```python
from build123d import *

# Parameters (mm, degrees)
BOSS_EXTRU_1_DEPTH                           = 6
ESQUISSE2_W                                  = 4
ESQUISSE2_H                                  = 4
BOSS_EXTRU_2_DEPTH                           = 4
TROU_POUR_TARAUDAGE_POUR_TROU_TARAUD_M2_D    = 1.6
TROU_POUR_TARAUDAGE_POUR_TROU_TARAUD_2_REACH = 15.115
TROU_POUR_TARAUDAGE_POUR_TROU_TARAUD_2_B_R   = 0.8
D_GAGEMENT_M31_D                             = 3.6


with BuildPart() as part:
    # Esquisse1 → Boss.-Extru.1 (new body)
    with BuildSketch(Plane.XY):
        Polygon((-10, 4), (10, 4), (10, 0), (7, 0), (7, -2), (2.2, -2), (2.2, 0), (-10, 0), align=None)
    extrude(amount=-BOSS_EXTRU_1_DEPTH)

    # Esquisse2 → Boss.-Extru.2 (add)
    with BuildSketch(Plane.XY):
        with Locations((-8, 2)):
            Rectangle(ESQUISSE2_W, ESQUISSE2_H)
        with Locations((8, 2)):
            Rectangle(ESQUISSE2_W, ESQUISSE2_H)
    extrude(amount=BOSS_EXTRU_2_DEPTH)

    # Trou pour taraudage pour trou taraud_ M2 (through all)
    with Locations(Plane(origin=(10, 0, 0), x_dir=(0, 0, -1), z_dir=(1, 0, 0))):
        with Locations((-2, 2)):
            Hole(TROU_POUR_TARAUDAGE_POUR_TROU_TARAUD_M2_D / 2)

    # Trou pour taraudage pour trou taraud 2 b → Trou pour taraudage pour trou taraud 2 (cut, up to next)
    with BuildSketch(Plane(origin=(0, 4, 0), x_dir=(1, 0, 0), z_dir=(0, 1, 0)), mode=Mode.PRIVATE) as trou_pour_taraudage_pour_trou_taraud_2_sk1:
        with Locations((-8, -2)):
            Circle(TROU_POUR_TARAUDAGE_POUR_TROU_TARAUD_2_B_R)
    trou_pour_taraudage_pour_trou_taraud_2_tool1 = extrude(trou_pour_taraudage_pour_trou_taraud_2_sk1.sketch, amount=-TROU_POUR_TARAUDAGE_POUR_TROU_TARAUD_2_REACH, mode=Mode.PRIVATE) & part.part
    add(trou_pour_taraudage_pour_trou_taraud_2_tool1.solids().sort_by_distance((-8, 4, 2))[0], mode=Mode.SUBTRACT)

    # Dégagement M31 (through all)
    with Locations(Plane(origin=(0, 4, 0), x_dir=(1, 0, 0), z_dir=(0, 1, 0))):
        with Locations((4.6, 3)):
            Hole(D_GAGEMENT_M31_D / 2)


solid = part.part
```
Geometry check sheet. Reference: the model listing, model coordinates, mm. A direction names the side the tool comes from. Give positions to 0.01 mm unless a question says otherwise; leave off trailing zeros. Order: outer loops, then holes, each group sorted by start corner. A loop starts at its lowest first (then second) coordinate and runs counter-clockwise, first axis right, second up.
1. Section check D-D, the plane x = 4.6. Enter the section's corners in (y, z), and give its area (3 significant figures).
2. Access from +Z, -Z, +X, -X, +Y, -Y to the whole of each face (thin tool, end or side, straight path). Record for faces 1 (the face through (-5, 0, -2)), 2 (the face through (7, -1, -3)), 3 (the face through (-7.57, 3.236, 1.325)), 4 (the face through (0, 2, -6)), 5 (the face through (6, 3, 2)).
3. Section check B-B, the plane z = 0.5. Enter the section's corners in (x, y), and give its area (3 significant figures).
4. Release check for a two-part mould opening along X. For faces 6 (the face through (8, 2, 4)), 7 (the face through (1, 2, 0)), 8 (the face through (10, 2, -1)) record: pulls with the +X half, pulls with the -X half, needs draft (parallel to the pull), parting line crosses it, or undercut.
5. Thickness scan on L1, parallel to Z at x = 4.6, y = 0.9; L2, parallel to X at y = 3.2, z = 2.5; L3, parallel to Z at x = -8.8, y = 2. Record the ranges inside material, lowest first.
6. Section check C-C, the plane x = -7. Enter the section's corners in (y, z), and give its area (3 significant figures).
7. Gauge pin test, flat ends, axial feed: pin 1 Ø5 at (x, z) = (-2.5, 0) entering from -Y; pin 2 Ø1.8 at (x, y) = (-2.5, 0.5) entering from +Z; pin 3 Ø1.6 at (y, z) = (-1.5, -4.5) entering from +X. Record the tip position at first contact, or that the pin passes through.
8. Section check A-A, the plane y = 3.3. Enter the section's corners in (x, z), and give its area (3 significant figures).
Values follow:
1. outline: (-2, -6) - (4, -6) - (4, -4.8) - (-2, -4.8) - close; (-2, -1.2) - (4, -1.2) - (4, 0) - (-2, 0) - close
1. area: 14.4 mm2
2. face 1: +Z, -Z, -X, -Y
2. face 2: +Z, -Z, +X, -Y
2. face 3: +Y
2. face 4: -Z, +X, -X, +Y, -Y
2. face 5: +Z, +Y, -Y
3. outline: (-10, 0) - (-6, 0) - (-6, 4) - (-10, 4) - close; (6, 0) - (10, 0) - (10, 4) - (6, 4) - close
3. area: 32.0 mm2
4. face 6: needs draft
4. face 7: undercut
4. face 8: pulls with the +X half
5. L1: z = -6 to -4.8, -1.2 to 0
5. L2: x = -10 to -8.62, -7.38 to -6, 6 to 10
5. L3: z = -6 to 1.2, 2.8 to 4
6. outline: (0, -6) - (4, -6) - (4, 4) - (0, 4) - close; hole circle Ø1.6 at (2, 2)
6. area: 38.0 mm2
7. pin 1: stops at y = 0
7. pin 2: stops at z = 0
7. pin 3: stops at x = 7
8. outline: (-10, -6) - (10, -6) - (10, 4) - (6, 4) - (6, 0) - (-6, 0) - (-6, 4) - (-10, 4) - close; hole circle Ø1.6 at (-8, 2); hole circle Ø3.6 at (4.6, -3)
8. area: 140 mm2
